Autodesk Inventor part; units mm, degrees
ref_plane "YZ Plane" through (0, 0, 0) normal (1, 0, 0) x (0, 1, 0)
ref_plane "XZ Plane" through (0, 0, 0) normal (0, 1, 0) x (-1, 0, 0)
ref_plane "XY Plane" through (0, 0, 0) normal (0, 0, 1) x (1, 0, 0)
sketch "Sketch1" plane through (0, 0, 0) normal (0, 1, 0) x (-1, 0, 0)
  line L0 (6.75, -3.8971) -> (0, -7.7942)
  line L1 (0, -7.7942) -> (-6.75, -3.8971)
  line L2 (-6.75, -3.8971) -> (-6.75, 3.8971)
  line L3 (-6.75, 3.8971) -> (0, 7.7942)
  line L4 (0, 7.7942) -> (6.75, 3.8971)
  line L5 (6.75, 3.8971) -> (6.75, -3.8971)
  circle A0 centre (0, 0) radius 3.5
  point P0 (-6.75, 0)
  point P1 (6.75, 0)
  dimension "d0" = 13.5
  dimension "d1" = 7
extrude "Extrusion1" add sketch "Sketch1" along normal blind 5.5
fillet "Fillet1" radius 0.254 20 edges at (3.375, 5.5, 5.8457) (-3.375, 5.5, 5.8457) (-6.75, 5.5, 0) (-3.375, 5.5, -5.8457) (3.375, 5.5, -5.8457) (6.75, 5.5, 0) (3.5, 5.5, 0) (3.5, 0, 0) (3.375, 0, 5.8457) (6.75, 0, 0) (3.375, 0, -5.8457) (-3.375, 0, -5.8457) (-6.75, 0, 0) (-3.375, 0, 5.8457) (6.75, 2.75, 3.8971) (6.75, 2.75, -3.8971) (0, 2.75, -7.7942) (-6.75, 2.75, -3.8971) (-6.75, 2.75, 3.8971) (0, 2.75, 7.7942)
properties part number "Threaded Rod Nut" material "Steel, Mild"
For this review, take the finished solid that the model builds, in its own axes (mm). Round coordinates to 2 decimals unless told otherwise and drop trailing zeros. Order: outer loops, then holes, each group sorted by start corner. A loop starts at its lowest first (then second) coordinate and runs counter-clockwise, first axis right, second up. Notation, with made-up numbers: (-15, 55.5) -> (20, 55.5) arc R22 cw to (20, 84.5) -> close; hole circle Ø3 at (47, 83.5). An arc over 180 degrees is marked (long way). Use a Markdown table: item, result.
Item 1: Take a section at A-A (z = 0). State the section outline as (x, y) points, plus the area to 3 significant figures.
Resolved:
| item | result |
|---|---|
| outline | (-6.75, 0.25) arc R0.25 ccw to (-6.5, 0) -> (-3.75, 0) arc R0.25 ccw to (-3.5, 0.25) -> (-3.5, 5.25) arc R0.25 ccw to (-3.75, 5.5) -> (-6.5, 5.5) arc R0.25 ccw to (-6.75, 5.25) -> close; (3.5, 0.25) arc R0.25 ccw to (3.75, 0) -> (6.5, 0) arc R0.25 ccw to (6.75, 0.25) -> (6.75, 5.25) arc R0.25 ccw to (6.5, 5.5) -> (3.75, 5.5) arc R0.25 ccw to (3.5, 5.25) -> close |
| area | 35.6 mm² |
Item 2: Take a section at B-B (y = 4.55). State the section outline as (x, z) points, plus the area to 3 significant figures.
Resolved:
| item | result |
|---|---|
| outline | (-6.75, -3.75) arc R0.25 ccw to (-6.62, -3.97) -> (-0.13, -7.72) arc R0.25 ccw to (0.13, -7.72) -> (6.62, -3.97) arc R0.25 ccw to (6.75, -3.75) -> (6.75, 3.75) arc R0.25 ccw to (6.62, 3.97) -> (0.13, 7.72) arc R0.25 ccw to (-0.13, 7.72) -> (-6.62, 3.97) arc R0.25 ccw to (-6.75, 3.75) -> close; hole circle Ø7 at (0, 0) |
| area | 119 mm² |
Item 3: Draft analysis for pull direction Z (two halves, no side actions). For faces 1 (the cylindrical face through (-3.233, 2.715, 1.341)), 2 (the flat face through (-3.33, 2.72, 5.87)), 3 (the flat face through (3, 0, -3)), 4 (the cylindrical face through (-3.291, 0.072, -5.806)), state which applies: +Z half, -Z half, draft (parallel to the pull), parting line (faces both ways), or undercut.
Resolved:
| item | result |
|---|---|
| face 1 | undercut |
| face 2 | +Z half |
| face 3 | draft |
| face 4 | -Z half |
Item 4: For pin 1 (3 mm diameter, centred on x = -2, y = 4, fed in from +Z), flat-tipped, find the tip position at first contact; note if it passes through.
Resolved:
| item | result |
|---|---|
| pin 1 | stops at z = 7.51 |
Item 5: For line 1 along Z through (x, y) = (0, 4); line 2 along Z through (x, y) = (2.5, 0.35); line 3 along X through (y, z) = (5.3, 1.5), list the stretches that pass through material, from the lowest coordinate up. Write a range as [from, to].
Resolved:
| item | result |
|---|---|
| line 1 | z = [-7.75, -3.5], [3.5, 7.75] |
| line 2 | z = [-6.35, -2.45], [2.45, 6.35] |
| line 3 | x = [-6.74, -3.17], [3.17, 6.74] |
